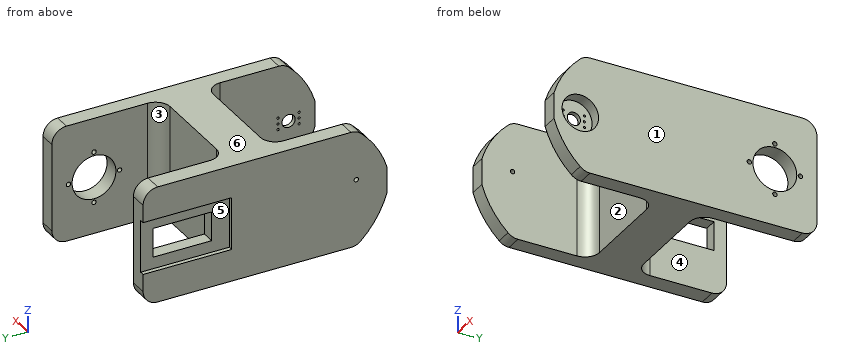
```python
from build123d import *

# Parameters (mm, degrees)
SKETCH1_W           = 80
SKETCH1_H           = 180
BOSS_EXTRUDE1_DEPTH = 100
SKETCH2_W           = 78.07363092
SKETCH2_H           = 74.951044638
CUT_EXTRUDE1_DEPTH  = 90
SKETCH3_R           = 12.5
CUT_EXTRUDE2_DEPTH  = 8
SKETCH4_R           = 0.75
CUT_EXTRUDE3_DEPTH  = 8
SKETCH5_R           = 1.5
CUT_EXTRUDE4_DEPTH  = 18
CUT_EXTRUDE5_DEPTH  = 110
SKETCH8_W           = 78.07363092
SKETCH8_H           = 150.808878852
CUT_EXTRUDE7_DEPTH  = 110
SKETCH12_W          = 80
SKETCH12_H          = 75.404439426
BOSS_EXTRUDE2_DEPTH = 1
SKETCH13_W          = 20
SKETCH13_H          = 40
CUT_EXTRUDE9_DEPTH  = 18
SKETCH14_W          = 36.018811194
SKETCH14_H          = 61.676046566
CUT_EXTRUDE10_DEPTH = 3
SKETCH15_W          = 80
SKETCH15_H          = 13.072149311
CUT_EXTRUDE11_DEPTH = 30
SKETCH16_R          = 15
CUT_EXTRUDE12_DEPTH = 30
SKETCH17_R          = 1.5
CUT_EXTRUDE13_DEPTH = 13
FILLET1_R           = 10
FILLET2_R           = 10
FILLET3_R           = 10


with BuildPart() as part:
    # Sketch1 → Boss-Extrude1 (new body)
    with BuildSketch(Plane(origin=(0, 0, 0), x_dir=(0, 0, -1), z_dir=(1, 0, 0))):
        Rectangle(SKETCH1_W, SKETCH1_H)
    extrude(amount=BOSS_EXTRUDE1_DEPTH)

    # Sketch2 → Cut-Extrude1 (cut)
    with BuildSketch(Plane.XY.offset(40)):
        with Locations((50, -52.524477681)):
            Rectangle(SKETCH2_W, SKETCH2_H)
    extrude(amount=-CUT_EXTRUDE1_DEPTH, mode=Mode.SUBTRACT)

    # Sketch3 → Cut-Extrude2 (cut)
    with BuildSketch(Plane(origin=(100, 0, 0), x_dir=(0, 0, -1), z_dir=(1, 0, 0))):
        with Locations((0, -72)):
            Circle(SKETCH3_R)
    extrude(amount=-CUT_EXTRUDE2_DEPTH, mode=Mode.SUBTRACT)

    # Sketch4 → Cut-Extrude3 (cut)
    with BuildSketch(Plane.ZY.offset(-89.03681546)):
        with BuildLine():
            ThreePointArc((-4.5, -72), (0, -76.5), (4.5, -72))
            Line((4.5, -72), (-4.5, -72))
        make_face()
        with BuildLine():
            Line((-4.5, -72), (4.5, -72))
            ThreePointArc((4.5, -72), (0, -67.5), (-4.5, -72))
        make_face()
        with Locations(Location((-4, -64.75, 0), (0, 0, 270))):
            Circle(SKETCH4_R)
        with Locations(Location((0, -64.75, 0), (0, 0, 270))):
            Circle(SKETCH4_R)
        with Locations(Location((4, -64.75, 0), (0, 0, 270))):
            Circle(SKETCH4_R)
        with Locations(Location((4, -79.25, 0), (0, 0, 270))):
            Circle(SKETCH4_R)
        with Locations(Location((0, -79.25, 0), (0, 0, 270))):
            Circle(SKETCH4_R)
        with Locations(Location((-4, -79.25, 0), (0, 0, 270))):
            Circle(SKETCH4_R)
    extrude(amount=-CUT_EXTRUDE3_DEPTH, mode=Mode.SUBTRACT)

    # Sketch5 → Cut-Extrude4 (cut)
    with BuildSketch(Plane.ZY):
        with Locations((6.03, -69)):
            Circle(SKETCH5_R)
    extrude(amount=-CUT_EXTRUDE4_DEPTH, mode=Mode.SUBTRACT)

    # Sketch6 → Cut-Extrude5 (cut)
    with BuildSketch(Plane(origin=(100, 0, 0), x_dir=(0, 0, -1), z_dir=(1, 0, 0))):
        with BuildLine():
            Line((40, -69.065791889), (40, -90))
            Line((40, -90), (8.943223126, -90))
            ThreePointArc((8.943223126, -90), (26.043708831, -81.865168262), (40, -69.065791889))
        make_face()
        with BuildLine():
            Line((-40, -69.065791889), (-40, -90))
            Line((-40, -90), (-8.943223126, -90))
            ThreePointArc((-8.943223126, -90), (-26.043708831, -81.865168262), (-40, -69.065791889))
        make_face()
    extrude(amount=-CUT_EXTRUDE5_DEPTH, mode=Mode.SUBTRACT)

    # Sketch8 → Cut-Extrude7 (cut)
    with BuildSketch(Plane.XY.offset(40)):
        with Locations((50, 90)):
            Rectangle(SKETCH8_W, SKETCH8_H)
    extrude(amount=-CUT_EXTRUDE7_DEPTH, mode=Mode.SUBTRACT)

    # Sketch12 → Boss-Extrude2 (add)
    with BuildSketch(Plane(origin=(10.96318454, 0, 0), x_dir=(0, 0, -1), z_dir=(1, 0, 0))):
        with Locations((0, 52.297780287)):
            Rectangle(SKETCH12_W, SKETCH12_H)
    extrude(amount=BOSS_EXTRUDE2_DEPTH)

    # Sketch13 → Cut-Extrude9 (cut)
    with BuildSketch(Plane.ZY):
        with Locations((0, 48.337059594)):
            Rectangle(SKETCH13_W, SKETCH13_H)
    extrude(amount=-CUT_EXTRUDE9_DEPTH, mode=Mode.SUBTRACT)

    # Sketch14 → Cut-Extrude10 (cut)
    with BuildSketch(Plane.ZY):
        with Locations((0, 47.120499576)):
            Rectangle(SKETCH14_W, SKETCH14_H)
    extrude(amount=-CUT_EXTRUDE10_DEPTH, mode=Mode.SUBTRACT)

    # Sketch15 → Cut-Extrude11 (cut)
    with BuildSketch(Plane(origin=(11.96318454, 0, 0), x_dir=(0, 0, -1), z_dir=(1, 0, 0))):
        with Locations((0, 83.463925345)):
            Rectangle(SKETCH15_W, SKETCH15_H)
    extrude(amount=-CUT_EXTRUDE11_DEPTH, mode=Mode.SUBTRACT)

    # Sketch16 → Cut-Extrude12 (cut)
    with BuildSketch(Plane(origin=(100, 0, 0), x_dir=(0, 0, -1), z_dir=(1, 0, 0))):
        with Locations((0.94, 61.16)):
            Circle(SKETCH16_R)
    extrude(amount=-CUT_EXTRUDE12_DEPTH, mode=Mode.SUBTRACT)

    # Sketch17 → Cut-Extrude13 (cut)
    with BuildSketch(Plane(origin=(100, 0, 0), x_dir=(0, 0, -1), z_dir=(1, 0, 0))):
        with Locations((0.94, 78.66)):
            Circle(SKETCH17_R)
        with Locations((18.44, 61.16)):
            Circle(SKETCH17_R)
        with Locations((0.94, 43.66)):
            Circle(SKETCH17_R)
        with Locations((-16.56, 61.16)):
            Circle(SKETCH17_R)
    extrude(amount=-CUT_EXTRUDE13_DEPTH, mode=Mode.SUBTRACT)

    # Fillet1
    fillet1_edges = [part.edges().sort_by_distance(p)[0] for p in [
        (89.03681546, 14.595560574, 0),
        (11.96318454, 14.595560574, 0),
        (89.03681546, -15.048955362, 0),
        (10.96318454, -15.048955362, 0),
    ]]
    fillet(fillet1_edges, radius=FILLET1_R)

    # Fillet2
    fillet2_edges = [part.edges().sort_by_distance(p)[0] for p in [
        (5.98159227, 76.927850689, 40),
        (5.98159227, 76.927850689, -40),
        (94.51840773, 90, 40),
        (94.51840773, 90, -40),
    ]]
    fillet(fillet2_edges, radius=FILLET2_R)

    # Fillet3
    fillet3_edges = [part.edges().sort_by_distance(p)[0] for p in [
        (94.51840773, -69.065791889, 40),
        (5.48159227, -69.065791889, 40),
        (94.51840773, -69.065791889, -40),
        (5.48159227, -69.065791889, -40),
    ]]
    fillet(fillet3_edges, radius=FILLET3_R)


solid = part.part
```
Could you check a few things on this model? Use its own coordinates, in mm. Face numbers are marked on the shaded views. A direction names the side the tool comes from. Round coordinates to 2 decimals unless told otherwise and drop trailing zeros. Loops run counter-clockwise (first coordinate to the right, second up) from the corner with the lowest first, then second, coordinate; pieces in that order, holes last.
Q1. For P1, Ø1.2, axis at y = -64.75, z = 0, coming from the +X side; P2, Ø8, axis at x = 41.5, z = -0.5, coming from the -Y side; P3, Ø2.5, axis at y = -64.75, z = -4, coming from the +X side, each with a flat end and sliding along its axis, tell me the tip position at first contact or that it passes through.
Q2. I want a section at A-A (y = 26.5). Write out the boundary of the cut face in (x, z), and give its area (3 significant figures).
Q3. I want a section at B-B (x = 35.5). Write out the boundary of the cut face in (y, z).
Q4. Please list where these lines run through material, in increasing order: L1, parallel to Z at x = 90, y = -64.75; L2, parallel to Y at x = 96.5, z = -0.94; L3, parallel to Y at x = 10.5, z = -7.
Q5. Thinking about a two-plate mould opening in X: for the marked faces 4, 5 and 6, which applies, pulls with the +X half, pulls with the -X half, needs draft (parallel to the pull), parting line crosses it, or undercut?
Q6. I want a section at C-C (x = 86.5). Write out the boundary of the cut face in (y, z), and give its area (3 significant figures).
Q7. On a 3-axis mill with a long thin cutter (end or side, diameter ignored), from which of +Z, -Z, +X, -X, +Y, -Y can I reach the whole of each face in a straight line? I mean the marked faces 1, 2 and 3. Say none if no direction works.
Answer below:
1. P1: stops at x = 10.96
1. P2: stops at y = -15.05
1. P3: stops at x = 92
2. outline: (0, -40) - (11.96, -40) - (11.96, 40) - (0, 40) - (0, 18.01) - (3, 18.01) - (3, -18.01) - (0, -18.01) - close; (89.04, -40) - (100, -40) - (100, 40) - (89.04, 40) - close
2. area: 1,730 mm2
3. outline: (-15.05, -40) - (14.6, -40) - (14.6, 40) - (-15.05, 40) - close
4. L1: z = -40 to -4.75, -3.25 to -0.75, 0.75 to 3.25, 4.75 to 40
4. L2: y = -90 to -84.46, -59.54 to 42.16, 45.16 to 46.16, 76.16 to 77.16, 80.16 to 90
4. L3: y = -90 to 28.34, 68.34 to 76.93
5. face 4: undercut
5. face 5: pulls with the -X half
5. face 6: needs draft
6. outline: (-18.39, -40) - (17.94, -40) - (17.94, 40) - (-18.39, 40) - close
6. area: 2,910 mm2
7. face 1: +Z, -Z, +X, +Y, -Y
7. face 2: +Z, -Z, -Y
7. face 3: +Z, -Z, +Y
